Read the model definition and answer for the solid it produces. Units are mm, in the model's axes. Face numbers are marked on the shaded views. A direction names the side the tool comes from. Coordinates: 2 decimals unless noted, no trailing zeros. Order: outer loops, then holes, each group sorted by start corner. A loop starts at its lowest first (then second) coordinate and runs counter-clockwise, first axis right, second up. Notation, with made-up numbers: M 12,7 L 41,7 A23 cw 41,42 Z; hole C 57,-3.75 d4. An arc over 180 degrees is marked long. Put each result on its own line as item: value.
from build123d import *

# Parameters (mm, degrees)
F0_W      = 30
F0_H      = 30
F1_DEPTH  = 30
F2_W      = 20
F2_H      = 20
F3_DEPTH  = 30.001
F5_DEPTH  = 5
F6_R      = 10
F7_DEPTH  = 5
F8_R      = 10
F9_DEPTH  = 5
F10_R     = 10
F11_DEPTH = 5


with BuildPart() as f1:
    # F0 (on Right) → F1 (new body)
    with BuildSketch(Plane.YZ):
        Rectangle(F0_W, F0_H)
    extrude(amount=F1_DEPTH)

    # F2 (on face) → F3 (cut, through all)
    with BuildSketch(Plane.YZ.offset(30)):
        Rectangle(F2_W, F2_H)
    extrude(amount=-F3_DEPTH, mode=Mode.SUBTRACT)

    # F4 (on face) → F5 (cut, through all)
    with BuildSketch(Plane.XZ.offset(15)):
        with BuildLine():
            Line((20, 5), (23.6602540378, 5))
            ThreePointArc((23.6602540378, 5), (22.0710678119, 7.0710678119), (20, 8.6602540378))
            Line((20, 8.6602540378), (20, 5))
        make_face()
        with BuildLine():
            Line((20, 5), (20, 8.6602540378))
            ThreePointArc((20, 8.6602540378), (12.411809549, 9.6592582629), (6.3397459622, 5))
            Line((6.3397459622, 5), (20, 5))
        make_face()
        with BuildLine():
            ThreePointArc((6.3397459622, 5), (7.9289321881, -7.0710678119), (20, -8.6602540378))
            Line((20, -8.6602540378), (20, 5))
            Line((20, 5), (6.3397459622, 5))
        make_face()
        with BuildLine():
            ThreePointArc((20, -8.6602540378), (23.6602540378, -5), (25, 0))
            ThreePointArc((25, 0), (24.6592582629, 2.588190451), (23.6602540378, 5))
            Line((23.6602540378, 5), (20, 5))
            Line((20, 5), (20, -8.6602540378))
        make_face()
    extrude(amount=-F5_DEPTH, mode=Mode.SUBTRACT)

    # F6 (on face) → F7 (cut, through all)
    with BuildSketch(Plane.XY.offset(15)):
        with Locations((15, 0)):
            Circle(F6_R)
    extrude(amount=-F7_DEPTH, mode=Mode.SUBTRACT)

    # F8 (on face) → F9 (cut, through all)
    with BuildSketch(Plane(origin=(0, 15, 0), x_dir=(-1, 0, 0), z_dir=(0, 1, 0))):
        with Locations((-15, 0)):
            Circle(F8_R)
    extrude(amount=-F9_DEPTH, mode=Mode.SUBTRACT)

    # F10 (on face) → F11 (cut, through all)
    with BuildSketch(Plane(origin=(0, 0, -15), x_dir=(1, 0, 0), z_dir=(0, 0, -1))):
        with Locations((15, 0)):
            Circle(F10_R)
    extrude(amount=-F11_DEPTH, mode=Mode.SUBTRACT)


solid = f1.part
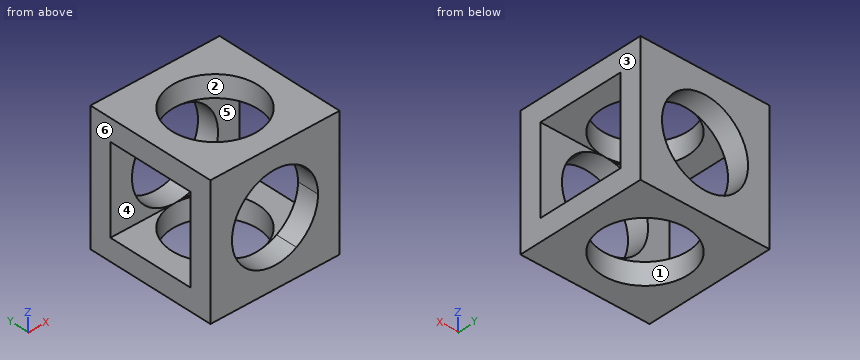
Q1. Find section B-B on z = -5.75. Write down the section's boundary in (x, y), plus the area to 3 significant figures.
Answers below:
outline: M 0,-15 L 6.82,-15 L 6.82,-10 L 0,-10 Z; M 0,10 L 6.82,10 L 6.82,15 L 0,15 Z; M 23.18,-15 L 30,-15 L 30,-10 L 23.18,-10 Z; M 23.18,10 L 30,10 L 30,15 L 23.18,15 Z
area: 136 mm^2
Q2. Find section D-D on x = 8.5. Write down the section's boundary in (y, z).
Answers below:
outline: M -15,-15 L -7.6,-15 L -7.6,-10 L -10,-10 L -10,-7.6 L -15,-7.6 Z; M -15,7.6 L -10,7.6 L -10,10 L -7.6,10 L -7.6,15 L -15,15 Z; M 7.6,-15 L 15,-15 L 15,-7.6 L 10,-7.6 L 10,-10 L 7.6,-10 Z; M 7.6,10 L 10,10 L 10,7.6 L 15,7.6 L 15,15 L 7.6,15 Z
Q3. Find section A-A on y = 0. Write down the section's boundary in (x, z), plus the area to 3 significant figures.
Answers below:
outline: M 0,-15 L 5,-15 L 5,-10 L 0,-10 Z; M 0,10 L 5,10 L 5,15 L 0,15 Z; M 25,-15 L 30,-15 L 30,-10 L 25,-10 Z; M 25,10 L 30,10 L 30,15 L 25,15 Z
area: 100 mm^2
Q4. Find section C-C on x = 15.75. Give the number of separate pieces and of enclosed holes in the cut face, plus the area to 3 significant figures.
Answers below:
separate pieces: 4
enclosed holes: 0
area: 101 mm^2
Q5. Consider line 1 along Z through (x, y) = (6.5, 9); line 2 along Z through (x, y) = (10, 10.5). Determine where each line is inside the solid, lowest interval first.
Answers below:
line 1: z = -15 to -10, 10 to 15
line 2: z = -15 to -8.66, 8.66 to 15
Q6. For a pull along X with two mould halves and no side action, classify the marked faces 1, 2, 3 and 4 as +X half, -X half, draft (parallel to the pull), parting line (faces both ways), or undercut.
Answers below:
face 1: undercut
face 2: undercut
face 3: +X half
face 4: draft
Q7. A tool of negligible diameter and unlimited length cuts with its end or side. For the marked faces 5 and 6, from which of +Z, -Z, +X, -X, +Y, -Y can it reach the whole face along a straight path? Write none if from no direction.
Answers below:
face 5: +X, -X
face 6: +Z, -Z, -X, +Y, -Y
